Geometry: final body of the model. Coordinates: model frame, mm. Face numbers are marked on the shaded views. Coordinates: 2 decimals unless noted, no trailing zeros. Order: outer loops, then holes, each group sorted by start corner. A loop starts at its lowest first (then second) coordinate and runs counter-clockwise, first axis right, second up. Notation, with made-up numbers: (46.5, 38.5) - (91.5, 38.5) arc R21 cw to (91.5, 69.5) - close; hole circle Ø3 at (29, -25.5). An arc over 180 degrees is marked (long way). Use a Markdown table: item, result. Add a question column.
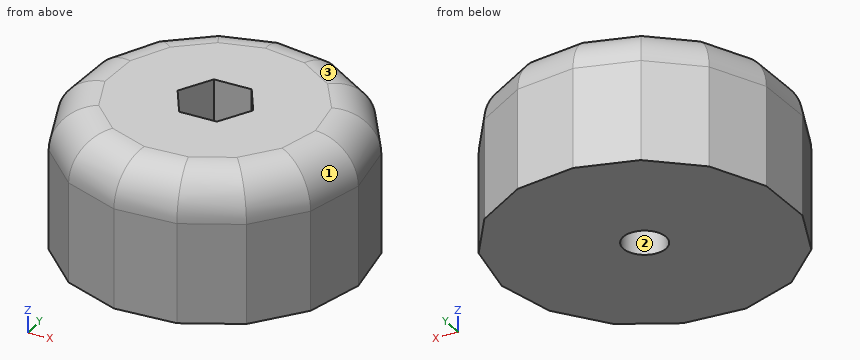
```python
from build123d import *

# Parameters (mm, degrees)
F1_DEPTH = 25.4
F2_R     = 7.62
F4_DEPTH = 12.7
F5_R     = 3.81
F6_DEPTH = 25.4


with BuildPart() as f1:
    # F0 (on Top) → F1 (new body)
    with BuildSketch(Plane.XY):
        Polygon((6.572324, -25.121964), (16.22214, -20.276851), (23.067001, -11.925686), (25.923367, -1.512462), (24.297348, 9.162281), (18.470097, 18.252782), (9.449198, 24.187211), (-1.205553, 25.939452), (-11.651853, 23.206526), (-20.083442, 16.46098), (-25.042421, 6.869182), (-25.671338, -3.91036), (-21.861448, -14.013766), (-14.271514, -21.694064), (-4.213906, -25.623261), align=None)
    extrude(amount=F1_DEPTH)

    # F2
    f2_edges = [f1.edges().sort_by_distance(p)[0] for p in [
        (-18.066481, -17.853915, 25.4),
        (-9.24271, -23.658662, 25.4),
        (1.179209, -25.372613, 25.4),
        (11.397232, -22.699407, 25.4),
        (19.644571, -16.101268, 25.4),
        (24.495184, -6.719074, 25.4),
        (25.110358, 3.82491, 25.4),
        (21.383722, 13.707531, 25.4),
        (13.959647, 21.219996, 25.4),
        (4.121822, 25.063331, 25.4),
        (-6.428703, 24.572989, 25.4),
        (-15.867648, 19.833753, 25.4),
        (-22.562932, 11.665081, 25.4),
        (-25.35688, 1.479411, 25.4),
        (-23.766393, -8.962063, 25.4),
    ]]
    fillet(f2_edges, radius=F2_R)

    # F3 (on face) → F4 (cut)
    with BuildSketch(Plane.XY.offset(25.4)):
        Polygon((-3.319764, -5.75), (3.319764, -5.75), (6.639528, 0), (3.319764, 5.75), (-3.319764, 5.75), (-6.639528, 0), align=None)
    extrude(amount=-F4_DEPTH, mode=Mode.SUBTRACT)

    # F5 (on face) → F6 (cut)
    with BuildSketch(Plane.XY.offset(12.7)):
        Circle(F5_R)
    extrude(amount=-F6_DEPTH, mode=Mode.SUBTRACT)


solid = f1.part
```
1) First-contact query: pin 1 (2 mm diameter, centred on x = 9, z = 21, fed in from +Y); pin 2 (5.5 mm diameter, centred on x = 1, z = 20.5, fed in from +Y); pin 3 (4 mm diameter, centred on x = 10, z = 11, fed in from -Y); pin 4 (3.5 mm diameter, centred on x = 1, y = -1, fed in from +Z). Flat tips, straight axial feed; report the tip coordinate or a pass-through.
2) Section query A-A (z = 5.5). Return the cut outline in (x, y), and give its area (3 significant figures).
3) Draft query along Y for the marked faces 1, 2 and 3. Return one class per face: released by +Y, released by -Y, zero draft, split by the parting line, or undercut.
4) Line query: line 1 (Y direction, x = 0, z = 7.75); line 2 (X direction, y = -1, z = 12); line 3 (X direction, y = 2, z = 13.5). Output: solid intervals per line, ascending. Write a range as from..to.
5) Section query B-B (z = 23.5). Return the cut outline in (x, y), and give its area (3 significant figures).
From the geometry:
| question | item | result |
|---|---|---|
| 1 | pin 1 | stops at y = 23.97 |
| 1 | pin 2 | stops at y = 25.86 |
| 1 | pin 3 | stops at y = -24.41 |
| 1 | pin 4 | passes through |
| 2 | outline | (-25.67, -3.91) - (-21.86, -14.01) - (-14.27, -21.69) - (-4.21, -25.62) - (6.57, -25.12) - (16.22, -20.28) - (23.07, -11.93) - (25.92, -1.51) - (24.3, 9.16) - (18.47, 18.25) - (9.45, 24.19) - (-1.21, 25.94) - (-11.65, 23.21) - (-20.08, 16.46) - (-25.04, 6.87) - close; hole circle Ø7.62 at (0, 0) |
| 2 | area | 2,010 mm^2 |
| 3 | face 1 | released by -Y |
| 3 | face 2 | undercut |
| 3 | face 3 | released by +Y |
| 4 | line 1 | y = -25.43..-3.81, 3.81..25.74 |
| 4 | line 2 | x = -25.5..-3.68, 3.68..25.85 |
| 4 | line 3 | x = -25.33..-5.48, 5.48..25.39 |
| 5 | outline | (-23.06, -3.51) - (-19.64, -12.59) - (-12.82, -19.49) - (-3.78, -23.02) - (5.9, -22.56) - (14.57, -18.21) - (20.72, -10.71) - (23.28, -1.36) - (21.82, 8.23) - (16.59, 16.39) - (8.49, 21.73) - (-1.08, 23.3) - (-10.47, 20.84) - (-18.04, 14.79) - (-22.49, 6.17) - close; hole (-6.64, 0) - (-3.32, -5.75) - (3.32, -5.75) - (6.64, 0) - (3.32, 5.75) - (-3.32, 5.75) - close |
| 5 | area | 1,550 mm^2 |
